Geometry: final body of the model. Coordinates: model frame, mm. Round coordinates to 2 decimals unless told otherwise and drop trailing zeros. Loops run counter-clockwise (first coordinate to the right, second up) from the corner with the lowest first, then second, coordinate; pieces in that order, holes last. Notation, with made-up numbers: M 83,14.25 L 90,14.25 A6 ccw 90,25.25 Z; hole C -11.5,-33.5 d3. An arc over 180 degrees is marked long. Answer as a JSON object with one key per item and string values.
```python
from build123d import *

# Parameters (mm, degrees)
F0_W           = 194.945
F0_H           = 44.45
F1_DEPTH       = 40.64
F2_D           = 5.1054
F2_DEPTH       = 25.4
F2_CSINK_D     = 9.525
F2_CSINK_ANGLE = 82
F2_TIP         = 1.5338169022
F3_R           = 7.14375
F5_DEPTH       = 194.946


with BuildPart() as f1:
    # F0 (on Front) → F1 (new body)
    with BuildSketch(Plane.XZ):
        with Locations((97.4725, 22.225)):
            Rectangle(F0_W, F0_H)
    extrude(amount=-F1_DEPTH)

    # F2
    with Locations(Plane.XZ):
        with Locations((16.51, 22.225), (178.435, 22.225)):
            CounterSinkHole(F2_D / 2, F2_CSINK_D / 2, depth=F2_DEPTH, counter_sink_angle=F2_CSINK_ANGLE)
            with Locations((0, 0, -(F2_DEPTH + F2_TIP / 2))):  # 118° drill point
                Cone(0, F2_D / 2, F2_TIP, mode=Mode.SUBTRACT)

    # F3
    f3_edges = [f1.edges().sort_by_distance(p)[0] for p in [
        (0, 20.32, 44.45),
        (194.945, 20.32, 44.45),
        (0, 20.32, 0),
        (194.945, 20.32, 0),
    ]]
    fillet(f3_edges, radius=F3_R)

    # F4 (on face) → F5 (cut, through all)
    with BuildSketch(Plane(origin=(0, 0, 0), x_dir=(0, -1, 0), z_dir=(-1, 0, 0))):
        with BuildLine():
            Line((-40.64, 7.14375), (-40.64, 22.225))
            Line((-40.64, 22.225), (-40.64, 37.30625))
            Line((-40.64, 37.30625), (-21.5269177657, 37.30625))
            ThreePointArc((-21.5269177657, 37.30625), (-94.615, 22.225), (-21.5269177657, 7.14375))
            Line((-21.5269177657, 7.14375), (-40.64, 7.14375))
        make_face()
        with BuildLine():
            Line((-40.64, 37.30625), (-40.64, 22.225))
            Line((-40.64, 22.225), (-18.415, 22.225))
            ThreePointArc((-18.415, 22.225), (-19.2010888332, 29.9244826732), (-21.5269177657, 37.30625))
            Line((-21.5269177657, 37.30625), (-40.64, 37.30625))
        make_face()
        with BuildLine():
            Line((-18.415, 22.225), (-40.64, 22.225))
            Line((-40.64, 22.225), (-40.64, 7.14375))
            Line((-40.64, 7.14375), (-21.5269177657, 7.14375))
            ThreePointArc((-21.5269177657, 7.14375), (-19.2010888332, 14.5255173268), (-18.415, 22.225))
        make_face()
    extrude(amount=-F5_DEPTH, mode=Mode.SUBTRACT)


solid = f1.part
```
1) Line query: probe 1 along Z at (x, y) = (16.51, 8.75); probe 2 along Y at (x, z) = (57, 29); probe 3 along X at (y, z) = (15.5, 37.5). Output: solid intervals per line, ascending.
Geometry results:
{"probe 1": "0 to 19.67, 24.78 to 44.45", "probe 2": "0 to 19.02", "probe 3": "0 to 194.94"}
2) First-contact query: pin 1 (6 mm diameter, centred on x = 86, z = 34.5, fed in from -Y); pin 2 (1 mm diameter, centred on y = 18, z = 5.5, fed in from +X); pin 3 (8 mm diameter, centred on x = 178.435, z = 22.225, fed in from -Y); pin 4 (1.5 mm diameter, centred on x = 58, z = 28, fed in from +Y). Flat tips, straight axial feed; report the tip coordinate or a pass-through.
Geometry results:
{"pin 1": "y = 0", "pin 2": "x = 194.85", "pin 3": "y = 0.88", "pin 4": "y = 18.98"}
3) Cut plane C-C on z = 30. Return the cut outline in (x, y) (3 decimals).
Geometry results:
{"outline": "M 0,0 L 194.945,0 L 194.945,19.217 L 0,19.217 Z"}
4) Cut plane B-B on x = 70. Return the cut outline in (y, z) (3 decimals), and give its area (3 significant figures).
Geometry results:
{"outline": "M 0,0 L 25.569,0 A38.1 cw 25.569,44.45 L 0,44.45 Z", "area": "920 mm2"}
5) Cut plane D-D on z = 14. Return the cut outline in (x, y) (3 decimals), and give its area (3 significant figures).
Geometry results:
{"outline": "M 0,0 L 194.945,0 L 194.945,19.313 L 0,19.313 Z", "area": "3,770 mm2"}
6) Pull-direction query (Z, two-part tool) for faces 1 (the face through (96, 13, 44.45)), 2 (the face through (0, 11, 22)), 3 (the face through (14.15, 10.63, 21.25)); classes: +Z half, -Z half, draft (parallel to the pull), parting line (faces both ways), or undercut.
Geometry results:
{"face 1": "+Z half", "face 2": "draft", "face 3": "undercut"}
